Input: part model. Units: mm. Frame: model coordinates. Give positions to 0.01 mm unless a question says otherwise; leave off trailing zeros. Loops run counter-clockwise (first coordinate to the right, second up) from the corner with the lowest first, then second, coordinate; pieces in that order, holes last. Notation, with made-up numbers: M 24,17 L 74,17 A29 ccw 74,41 Z; hole C 30.5,5.5 d6. An arc over 180 degrees is marked long. Answer as a JSON object with one key per item and string values. Group by question number.
1) Ray query, L1, parallel to Z at x = -490, y = 1.15; L2, parallel to Y at x = -368, z = -0.25. Return the intervals inside material, ascending.
2) First-contact query: P1, Ø0.5, axis at x = -252, z = -9.5, coming from the -Y side; P2, Ø0.8, axis at x = -237, y = 2.5, coming from the -Z side. Flat tips, straight axial feed; report the tip coordinate or a pass-through.
3) Section query A-A on x = -428. Return loops of the section in (y, z).
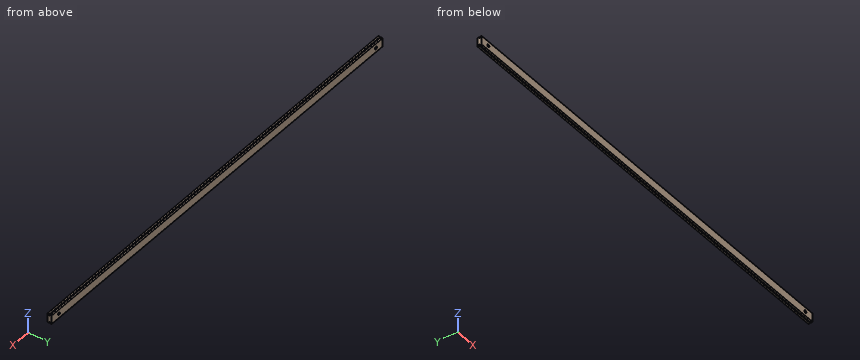
Autodesk Inventor part; units mm, degrees
ref_plane "YZ Plane" through (0, 0, 0) normal (1, 0, 0) x (0, 1, 0)
ref_plane "XZ Plane" through (0, 0, 0) normal (0, 1, 0) x (-1, 0, 0)
ref_plane "XY Plane" through (0, 0, 0) normal (0, 0, 1) x (1, 0, 0)
sketch "Sketch1" plane through (0, 0, 0) normal (0, 1, 0) x (-1, 0, 0)
  line L0 (0, 0) -> (0, -10)
  line L1 (0, -10) -> (500, -10)
  line L2 (500, -10) -> (500, 0)
  line L3 (500, 0) -> (0, 0)
  dimension "d0" = 10
  dimension "d1" = 500
  dimension "d2" = 500
extrude "Extrusion1" add sketch "Sketch1" along normal blind 5
sketch "Sketch5" plane through (0, 0, 0) normal (1, 0, 0) x (0, 0, -1)
  line L0 (1, 3) -> (0, 3)
  line L1 (0, 3) -> (0, 2)
  line L2 (0, 2) -> (1, 2)
  line L3 (1, 2) -> (1, 3)
  line L4 (10, 3) -> (9, 3)
  line L5 (9, 3) -> (9, 2)
  line L6 (9, 2) -> (10, 2)
  line L7 (10, 2) -> (10, 3)
  line L8 (10, 0) -> (10, 5)
  line L9 (0, 0) -> (0, 5)
  point P0 (10, 2.5)
  point P1 (0, 2.5)
  point P2 (10, 2.5)
  point P3 (0, 2.5)
  dimension "d33" = 1
  dimension "d34" = 1
  dimension "d35" = 1
  dimension "d36" = 1
  dimension "d37" = 1
  dimension "d38" = 1
  dimension "d39" = 1
extrude "Extrusion2" cut sketch "Sketch5" against normal up to next
sketch "Sketch7" plane through (0, 0, 0) normal (0, -1, 0) x (1, 0, 0)
  circle A0 centre (-11, -5) radius 1.5
  circle A1 centre (-490, -5) radius 1.5
  line L0 (-500, -10) -> (-500, 0)
  point P0 (0, 0)
  dimension "d42" = 3
  dimension "d43" = 3
  dimension "d44" = 479
  dimension "d45" = 10
extrude "Extrusion3" cut sketch "Sketch7" against normal up to next
sketch "Sketch2" plane through (0, 0, 0) normal (0, -1, 0) x (1, 0, 0)
  point P0 (-485, -5)
sketch "Sketch3" plane through (0, 0, 0) normal (0, -1, 0) x (1, 0, 0)
  point P0 (-15, -5)
properties part number "relsa2" material "Brass, Soft Yellow"
Output:
{
 "1": {"L1": "z = -10 to -6.5, -3.5 to 0", "L2": "y = 0 to 2, 3 to 5"},
 "2": {"P1": "stops at y = 0", "P2": "stops at z = -9"},
 "3": {"outline": "M 0,-10 L 2,-10 L 2,-9 L 3,-9 L 3,-10 L 5,-10 L 5,0 L 3,0 L 3,-1 L 2,-1 L 2,0 L 0,0 Z"}
}
